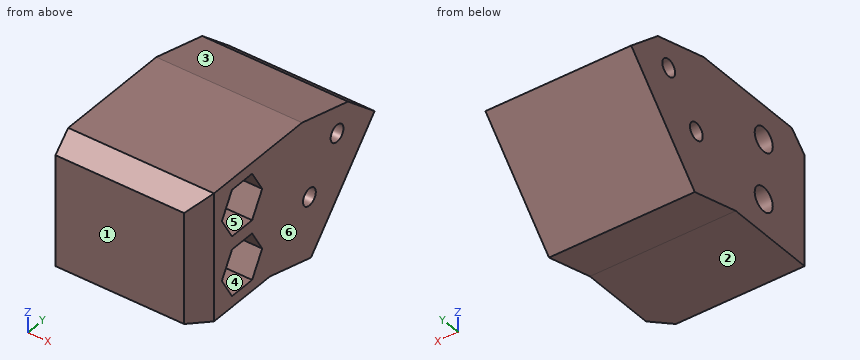
from build123d import *

# Parameters (mm, degrees)
SKETCH1_R           = 1
BOSS_EXTRUDE1_DEPTH = 17.05
CHAMFER3_SIZE       = 2
SKETCH4_R           = 1.411016709
CUT_EXTRUDE2_DEPTH  = 35.812450989
CUT_EXTRUDE3_DEPTH  = 35.812450989
CUT_EXTRUDE4_DEPTH  = 10


with BuildPart() as part:
    # Sketch1 → Boss-Extrude1 (new body)
    with BuildSketch(Plane(origin=(0, 0, 0), x_dir=(0, 0, -1), z_dir=(1, 0, 0))):
        Polygon((-7.5, 0), (7.5, 0), (7.5, 10.76), (9.149426619, 17.160897736), (-4.103828097, 28.939458123), (-7.5, 15.76), align=None)
        with Locations((-2.957491833, 21.231429279)):
            Circle(SKETCH1_R, mode=Mode.SUBTRACT)
        with Locations((1.901052893, 16.913496539)):
            Circle(SKETCH1_R, mode=Mode.SUBTRACT)
    extrude(amount=BOSS_EXTRUDE1_DEPTH)

    # Chamfer3
    chamfer3_edges = [part.edges().sort_by_distance(p)[0] for p in [
        (8.525, 0, 7.5),
        (17.05, 0, 0),
    ]]
    chamfer(chamfer3_edges, length=CHAMFER3_SIZE)

    # Sketch4 → Cut-Extrude2 (cut, through all)
    with BuildSketch(Plane(origin=(17.05, 0, 0), x_dir=(0, 0, -1), z_dir=(1, 0, 0))):
        with Locations((-3.500000028, 6.380001803)):
            Circle(SKETCH4_R)
        with Locations((3.5, 6.380001848)):
            Circle(SKETCH4_R)
    extrude(amount=-CUT_EXTRUDE2_DEPTH, mode=Mode.SUBTRACT)

    # Sketch5 → Cut-Extrude3 (cut, through all)
    with BuildSketch(Plane(origin=(17.05, 0, 0), x_dir=(0, 0, -1), z_dir=(1, 0, 0))):
        Polygon((-4.103828097, 28.939458123), (-2.03016404, 27.096531397), (-5.648400148, 22.945467464), align=None)
    extrude(amount=-CUT_EXTRUDE3_DEPTH, mode=Mode.SUBTRACT)

    # Sketch6 → Cut-Extrude4 (cut)
    with BuildSketch(Plane(origin=(17.05, 0, 0), x_dir=(0, 0, -1), z_dir=(1, 0, 0))):
        Polygon((-3.500000028, 3.230001803), (-0.772020006, 4.805001803), (-0.772020006, 7.955001803), (-3.500000028, 9.530001803), (-6.22798005, 7.955001803), (-6.22798005, 4.805001803), align=None)
        Polygon((6.22798005, 4.805001803), (3.500000028, 3.230001803), (0.772020006, 4.805001803), (0.772020006, 7.955001803), (3.500000028, 9.530001803), (6.22798005, 7.955001803), align=None)
    extrude(amount=-CUT_EXTRUDE4_DEPTH, mode=Mode.SUBTRACT)


solid = part.part
The listing builds one solid part. Answer for the finished solid, in the listing's coordinates (mm). Face numbers are marked on the shaded views. A direction names the side the tool comes from. Give positions to 0.01 mm unless a question says otherwise; leave off trailing zeros. Write each loop counter-clockwise with the first axis right and the second up, starting at its lowest first coordinate (ties: lowest second). Pieces come first, ordered by that corner, then holes.
1) Section A-A (x = 1.5) is taken. Write down the section's boundary in (y, z), and give its area (3 significant figures).
2) Section D-D (z = -8) is taken. Write down the section's boundary in (x, y).
3) Given P1, Ø2.5, axis at x = 11.5, y = 6.5, coming from the -Z side; P2, Ø1, axis at x = 5.5, z = -4, coming from the +Y side; P3, Ø1.7, axis at y = 6.38, z = -3.5, coming from the -X side; P4, Ø1.5, axis at x = 8, z = 5, coming from the +Y side, each flat-ended and moving along its own axis, determine where each tip first touches the part or whether it passes through.
4) Section C-C (x = 15.75) is taken. Write down the section's boundary in (y, z) (1 decimal).
5) Section B-B (y = 3.75) is taken. Write down the section's boundary in (x, z), and give its area (3 significant figures).
6) A tool of negligible diameter and unlimited length cuts with its end or side. For the marked faces 5 and 6, from which of +Z, -Z, +X, -X, +Y, -Y can it reach the whole face along a straight path? Write none if from no direction.
7) Find the intervals of material crossed by L1, parallel to Y at x = 6.75, z = 2.75; L2, parallel to Z at x = 12.25, y = 3.5; L3, parallel to Y at x = 3, z = 3.5, in increasing order.
8) For a pull along Z with two mould halves and no side action, classify the marked faces 1, 2, 3 and 4 as pulls with the +Z half, pulls with the -Z half, needs draft (parallel to the pull), parting line crosses it, or undercut.
Response:
1. outline: (0, -7.5) - (10.76, -7.5) - (17.16, -9.15) - (27.1, 2.03) - (22.95, 5.65) - (15.76, 7.5) - (2, 7.5) - (0, 5.5) - close; hole circle Ø2.82 at (6.38, -3.5); hole circle Ø2.82 at (6.38, 3.5); hole circle Ø2 at (16.91, -1.9); hole circle Ø2 at (21.23, 2.96)
1. area: 330 mm2
2. outline: (0, 12.7) - (17.05, 12.7) - (17.05, 18.18) - (0, 18.18) - close
3. P1: stops at z = -7.5
3. P2: stops at y = 22.18
3. P3: passes through
3. P4: stops at y = 24.55
4. outline: (0.7, -7.5) - (10.8, -7.5) - (17.2, -9.1) - (27.1, 2) - (22.9, 5.6) - (15.8, 7.5) - (2, 7.5) - (0.7, 6.2) - close; hole (3.2, -3.5) - (4.8, -6.2) - (8, -6.2) - (9.5, -3.5) - (8, -0.8) - (4.8, -0.8) - close; hole (3.2, 3.5) - (4.8, 0.8) - (8, 0.8) - (9.5, 3.5) - (8, 6.2) - (4.8, 6.2) - close; hole circle Ø2 at (16.9, -1.9); hole circle Ø2 at (21.2, 3)
5. outline: (0, -7.5) - (17.05, -7.5) - (17.05, -4.4) - (7.05, -4.4) - (7.05, -2.6) - (17.05, -2.6) - (17.05, 2.6) - (7.05, 2.6) - (7.05, 4.4) - (17.05, 4.4) - (17.05, 7.5) - (0, 7.5) - close
5. area: 220 mm2
6. face 5: +X
6. face 6: +Z, -Z, +X, +Y, -Y
7. L1: y = 0 to 5.18, 7.58 to 20.25, 22.21 to 26.27
7. L2: z = -7.5 to -3.97, -3.03 to 3.03, 3.97 to 7.5
7. L3: y = 0 to 4.97, 7.79 to 20.39, 22.07 to 25.41
8. face 1: needs draft
8. face 2: pulls with the -Z half
8. face 3: pulls with the +Z half
8. face 4: undercut
